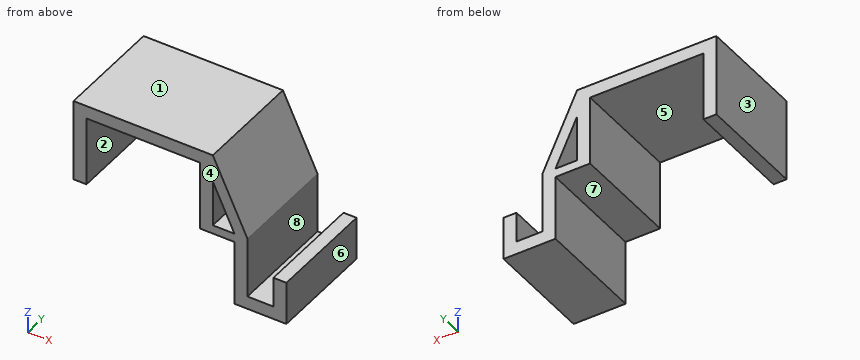
```python
from build123d import *

# Parameters (mm, degrees)
F0_W     = 3
F0_H     = 16
F0_H_2   = 3
F0_W_2   = 26.2
F0_H_3   = 7
F1_DEPTH = 25


with BuildPart() as f1:
    # F0 (on Front) → F1 (new body)
    with BuildSketch(Plane.XZ):
        with Locations((-14.6, 0)):
            Rectangle(F0_W, F0_H)
        with Locations((-14.6, 9.5)):
            Rectangle(F0_W, F0_H_2)
        with Locations((0, 9.5)):
            Rectangle(F0_W_2, F0_H_2)
        with Locations((14.6, 9.5)):
            Rectangle(F0_W, F0_H_2)
        Polygon((13.1, 8), (13.1, -8), (16.1, -8), (16.1, -6), (16.1, 4.625), (16.1, 8), align=None)
        Polygon((16.1, 11), (16.1, 8), (16.1, 4.625), (21.1, -6), (24.1, -6), align=None)
        Polygon((16.1, -6), (16.1, -8), (21.1, -8), (24.1, -8), (24.1, -6), (21.1, -6), align=None)
        Polygon((24.1, -8), (21.1, -8), (21.1, -23), (24.1, -23), (24.1, -20), align=None)
        Polygon((30.1, -20), (24.1, -20), (24.1, -23), (33.1, -23), (33.1, -20), align=None)
        with Locations((31.6, -16.5)):
            Rectangle(F0_W, F0_H_3)
    extrude(amount=F1_DEPTH)


solid = f1.part
```
Geometry: final body of the model. Coordinates: model frame, mm. Face numbers are marked on the shaded views. A direction names the side the tool comes from. Round coordinates to 2 decimals unless told otherwise and drop trailing zeros. Write each loop counter-clockwise with the first axis right and the second up, starting at its lowest first coordinate (ties: lowest second). Pieces come first, ordered by that corner, then holes. Notation, with made-up numbers: (39, 8.5) -> (61, 8.5) arc R20 ccw to (61, 47.5) -> close; hole circle Ø2 at (12, -20). An arc over 180 degrees is marked (long way). Return JSON: item names as keys, results as strings.
Q1. Ray query, line 1 (X direction, y = -19, z = -18); line 2 (X direction, y = -12.5, z = 3); line 3 (X direction, y = -4, z = 0). Return the intervals inside material, ascending.
From the geometry:
{"line 1": "21.1 to 24.1, 30.1 to 33.1", "line 2": "-16.1 to -13.1, 13.1 to 16.1, 16.86 to 19.86", "line 3": "-16.1 to -13.1, 13.1 to 16.1, 18.28 to 21.28"}
Q2. Set-up query: the marked faces 4, 5, 6, 7 and 8. Return all of +Z, -Z, +X, -X, +Y, -Y with unobstructed straight access to the full face (end or side cutting, diameter ignored); none if empty.
From the geometry:
{"face 4": "+Z, -Z, +X, -X, -Y", "face 5": "-Z, +Y, -Y", "face 6": "+Z, -Z, +X, +Y, -Y", "face 7": "-Z, -X, +Y, -Y", "face 8": "+Z, +Y, -Y"}
Q3. Section C-C on z = 2.5. Return the cut outline in (x, y), and give its area (3 significant figures).
From the geometry:
{"outline": "(-16.1, -25) -> (-13.1, -25) -> (-13.1, 0) -> (-16.1, 0) -> close; (13.1, -25) -> (16.1, -25) -> (16.1, 0) -> (13.1, 0) -> close; (17.1, -25) -> (20.1, -25) -> (20.1, 0) -> (17.1, 0) -> close", "area": "225 mm2"}
Q4. First-contact query: pin 1 Ø0.9 at (x, y) = (-15, -16.5) entering from -Z; pin 2 Ø1.5 at (x, y) = (32.5, -15.5) entering from +Z; pin 3 Ø5 at (y, z) = (-16, -1) entering from +X. Flat tips, straight axial feed; report the tip coordinate or a pass-through.
From the geometry:
{"pin 1": "z = -8", "pin 2": "z = -13", "pin 3": "x = 22.92"}
Q5. Section B-B on y = -12. Return the cut outline in (x, z) (3 decimals), and give its area (3 significant figures).
From the geometry:
{"outline": "(-16.1, -8) -> (-13.1, -8) -> (-13.1, 8) -> (13.1, 8) -> (13.1, -8) -> (21.1, -8) -> (21.1, -23) -> (33.1, -23) -> (33.1, -13) -> (30.1, -13) -> (30.1, -20) -> (24.1, -20) -> (24.1, -6) -> (16.1, 11) -> (-16.1, 11) -> close; hole (16.1, -6) -> (21.1, -6) -> (16.1, 4.625) -> close", "area": "343 mm2"}
Q6. Section D-D on x = 6.5. Return the cut outline in (y, z).
From the geometry:
{"outline": "(-25, 8) -> (0, 8) -> (0, 11) -> (-25, 11) -> close"}
Q7. Section A-A on z = -19. Return the cut outline in (x, y), and give its area (3 significant figures).
From the geometry:
{"outline": "(21.1, -25) -> (24.1, -25) -> (24.1, 0) -> (21.1, 0) -> close; (30.1, -25) -> (33.1, -25) -> (33.1, 0) -> (30.1, 0) -> close", "area": "150 mm2"}
Q8. Mould query, pull axis X, two halves, no side actions, for the marked faces 1, 2 and 3. Classes: +X half, -X half, draft (parallel to the pull), parting line (faces both ways), or undercut.
From the geometry:
{"face 1": "draft", "face 2": "undercut", "face 3": "-X half"}
